Source: CAD feature listing. Evaluate the final solid. Frame: model axes, mm. A direction names the side the tool comes from. Coordinates: 2 decimals unless noted, no trailing zeros. Order: outer loops, then holes, each group sorted by start corner. A loop starts at its lowest first (then second) coordinate and runs counter-clockwise, first axis right, second up.
Item 1: Ray query, line 1 (Y direction, x = -11, z = 0.05); line 2 (X direction, y = 10, z = -1.35); line 3 (Y direction, x = -16.6, z = 0). Return the intervals inside material, ascending.
Item 2: Mould query, pull axis Y, two halves, no side actions, for faces 4 (the cylindrical face through (-8.092, -10.737, 5.917)), 5 (the flat face through (13, 13.5, 0)), 6 (the flat face through (13, -13.5, 0)). Classes: released by +Y, released by -Y, zero draft, split by the parting line, or undercut.
Item 3: Section B-B on y = -3.5. Return the cut outline in (x, z) (3 decimals), then the cut area to 4 significant figures.
Item 4: Contact query for flat-ended pins moving along their axis: P1, Ø4.5, axis at x = 16.5, z = 0, coming from the +Y side; P2, Ø5, axis at x = 9, y = -10, coming from the +Z side (3 decimals); P3, Ø4.5, axis at x = -17, z = 0, coming from the -Y side. Output: stop coordinate, or through.
Item 5: Reachability of faces 1 (the flat face through (-9.1, -13.5, 7.4)), 2 (the flat face through (-4, -2.75, 6)), 3 (the flat face through (18, -4.75, 6)) from +Z, -Z, +X, -X, +Y, -Y: full face, straight path, thin tool, end or side. Return the list, or none.
Item 6: Section A-A on x = 9. Return the cut outline in (y, z) (3 decimals).
Autodesk Inventor part; units mm, degrees
ref_plane "Plan de construction1" through (-9.85, -13.5, 3) normal (0, 0, 1) x (1, 0, 0)
ref_plane "YZ Plane" through (0, 0, 0) normal (1, 0, 0) x (0, 1, 0)
ref_plane "XZ Plane" through (0, 0, 0) normal (0, 1, 0) x (-1, 0, 0)
sketch "Esquisse1" plane through (0, 0, 0) normal (0, 0, 1) x (1, 0, 0)
  line L0 (-21, -13.5) -> (21, -13.5)
  line L1 (21, -13.5) -> (21, 13.5)
  line L2 (21, 13.5) -> (-21, 13.5)
  line L3 (-21, 13.5) -> (-21, -13.5)
  line L4 (-21, -13.5) -> (21, 13.5) construction
  line L5 (21, -13.5) -> (-21, 13.5) construction
  point P0 (0, 0)
  dimension "d0" = 42
  dimension "d1" = 27
extrude "Extrusion1" add sketch "Esquisse1" along normal mid plane 5.75
sketch "Esquisse2" plane through (0, 0, 2.875) normal (0, 0, 1) x (1, 0, 0)
  line L0 (16, -4.75) -> (21, -4.75)
  line L1 (21, -4.75) -> (21, 4)
  line L2 (21, 4) -> (16, 4)
  line L3 (16, 4) -> (16, -4.75)
  line L4 (-21, 6) -> (21, 6)
  line L5 (21, 6) -> (21, 8)
  line L6 (21, 8) -> (-21, 8)
  line L7 (-21, 8) -> (-21, 6)
  line L8 (-21, -4.75) -> (13, -4.75)
  line L9 (13, -4.75) -> (13, -2.75)
  line L10 (13, -2.75) -> (-21, -2.75)
  line L11 (-21, -2.75) -> (-21, -4.75)
  line L12 (-21, -13.5) -> (21, -13.5) construction
  line L13 (21, -13.5) -> (21, 13.5) construction
  line L14 (21, 13.5) -> (-21, 13.5) construction
  line L15 (-21, 13.5) -> (-21, -13.5) construction
  point P0 (0, 0)
  dimension "d4" = 2
  dimension "d5" = 2
  dimension "d6" = 5
  dimension "d7" = 8.75
  dimension "d8" = 2
  dimension "d9" = 5.5
  dimension "d10" = 34
extrude "Extrusion2" add sketch "Esquisse2" along normal blind 6
sketch "Esquisse3" plane through (0, 0, 2.875) normal (0, 0, 1) x (1, 0, 0)
  line L0 (-9.85, 8) -> (7.55, 8)
  line L1 (7.55, 8) -> (7.55, 13.5)
  line L2 (7.55, 13.5) -> (-9.85, 13.5)
  line L3 (-9.85, 13.5) -> (-9.85, 8)
  line L4 (-21, 6) -> (21, 6) construction
  line L5 (21, 6) -> (21, 8) construction
  line L6 (21, 8) -> (-21, 8) construction
  line L7 (-21, 8) -> (-21, 6) construction
  line L8 (-21, 8) -> (21, 8) construction
  line L9 (21, 8) -> (21, 13.5) construction
  line L10 (21, 13.5) -> (-21, 13.5) construction
  line L11 (-21, 13.5) -> (-21, 8) construction
  line L12 (21, 8) -> (-21, 8) construction
  line L13 (-21, -13.5) -> (21, -13.5)
  line L14 (-9.85, -13.5) -> (7.55, -13.5)
  line L15 (7.55, -13.5) -> (7.55, -8.05)
  line L16 (7.55, -8.05) -> (-9.85, -8.05)
  line L17 (-9.85, -8.05) -> (-9.85, -13.5)
  line L18 (-21, -4.75) -> (13, -4.75)
  point P0 (0, 0)
  dimension "d13" = 17.4
  dimension "d14" = 11.15
  dimension "d17" = 3.3
extrude "Extrusion3" add sketch "Esquisse3" along normal up to surface (6 mm away)
ref_plane "Plan de construction1" through (-9.85, -13.5, 3) normal (0, 0, 1) x (1, 0, 0)
sketch "Esquisse5" plane through (-9.85, -13.5, 3) normal (0, 0, 1) x (1, 0, 0)
  line L0 (8.7, 27) -> (8.7, 37.7161)
  line L1 (0, 27) -> (17.4, 27)
  line L2 (0, 27) -> (6.45, 33.5)
  line L3 (6.45, 33.5) -> (8.7, 33.5)
  line L4 (0, 27) -> (8.7, 27)
  line L5 (-11.15, 27) -> (30.85, 27)
  point P0 (9.85, 13.5)
  dimension "d18" = 4.5
  dimension "d19" = 6.5
revolve "Révolution1" add sketch "Esquisse5" angle 360 about axis through (-1.15, 13.5, 3) along (0, 1, 0)
sketch "Esquisse7" plane through (-1.15, 20, 3) normal (0, 1, 0) x (1, 0, 0)
  circle A0 centre (0, 0) radius 2.25 construction
  point P0 (1.15, 3)
hole "Perçage1" at (-1.15, 20, 3) direction (0, -1, 0) diameter 2.459 depth 11 tip angle 118
mirror "Symétrie2" about plane through (0, 0, 0) normal (0, 1, 0) of "Révolution1", "Perçage1"
sketch "Esquisse6" plane through (0, 0, 0) normal (0, 1, 0) x (-1, 0, 0)
  line L0 (7.5667, 8.875) -> (-5.2667, 8.875)
  arc A0 (7.5667, 8.875) -> (-5.2667, 8.875) centre (1.15, 3) ccw
  line L1 (7.5667, -2.875) -> (-5.2667, -2.875)
  arc A1 (-5.2667, -2.875) -> (7.5667, -2.875) centre (1.15, 3) ccw
  point P0 (0, 0)
extrude "Extrusion4" cut sketch "Esquisse6" along normal through all both and the other way through all
sketch "Esquisse8" plane through (-21, -13.5, -2.875) normal (-1, 0, 0) x (0, 0, 1)
  point P0 (2.875, 13.5)
  point P1 (2.875, 13.5)
hole "Perçage2" at (-21, 0, 0) direction (1, 0, 0) diameter 2.459 depth 6 tip angle 118
sketch "Esquisse9" plane through (21, -13.5, -2.875) normal (1, 0, 0) x (0, 0, -1)
  line L0 (-11.75, 8.75) -> (-11.75, 17.5)
  line L1 (-5.75, 17.5) -> (-11.75, 17.5)
  point P0 (-2.875, 13.5)
  point P1 (-8.35, 13.95)
  dimension "d37" = 3.4
  dimension "d38" = 3.55
hole "Perçage3" at (21, 0.45, 5.475) direction (-1, 0, 0) diameter 2.459 end through all
sketch "Esquisse10" plane through (0, 0, -2.875) normal (0, 0, -1) x (-1, 0, 0)
  line L0 (21, -13.5) -> (21, 13.5)
  point P0 (0, 0)
  point P1 (-9, -10)
  point P2 (-9, 10)
  point P3 (11, 10)
  point P4 (11, -10)
  dimension "d46" = 20
  dimension "d47" = 20
  dimension "d48" = 10
  dimension "d49" = 10
hole "Perçage4" at (9, -10, -2.875) at (9, 10, -2.875) at (-11, 10, -2.875) at (-11, -10, -2.875) direction (0, 0, 1) diameter 3 end through all
sketch "Esquisse11" plane through (0, 0, -2.875) normal (0, 0, -1) x (-1, 0, 0)
  line L0 (21, -13.5) -> (21, 13.5)
  line L1 (21, 13.5) -> (7.5667, 13.5)
  point P0 (0, 0)
  point P1 (-5.5, 1.6)
  point P2 (12.75, 1.6)
  dimension "d57" = 18.25
  dimension "d58" = 8.25
  dimension "d59" = 11.9
hole "Perçage5" at (5.5, 1.6, -2.875) at (-12.75, 1.6, -2.875) direction (0, 0, 1) diameter 2.459 end through all
sketch "Esquisse12" plane through (-9.85, -8.05, 8.875) normal (0, 0, 1) x (1, 0, 0)
  arc A0 (17.4, -2.3341) -> (17.4, -1.5659) centre (18.85, -1.95) ccw construction
  arc A1 (0, -0.9869) -> (0, -2.9131) centre (-1.15, -1.95) ccw construction
  arc A2 (0, 19.0131) -> (0, 17.0869) centre (-1.15, 18.05) ccw construction
  arc A3 (17.4, 17.6659) -> (17.4, 18.4341) centre (18.85, 18.05) ccw construction
  circle A4 centre (18.85, -1.95) radius 3
  circle A5 centre (-1.15, -1.95) radius 1.5
  circle A6 centre (-1.15, -1.95) radius 3
  circle A7 centre (-1.15, 18.05) radius 3
  circle A8 centre (18.85, 18.05) radius 1.5
  circle A9 centre (18.85, 18.05) radius 3
  point P0 (9.85, 8.05)
  dimension "d67" = 6
  dimension "d68" = 6
  dimension "d69" = 6
  dimension "d70" = 6
extrude "Extrusion5" cut sketch "Esquisse12" against normal up to surface (6 mm away)
equation "\"d68\" = d67"
equation "\"d69\" = d67"
equation "\"d70\" = d68"
properties part number "Platine" material "Aluminium"
Answer list:
1. line 1: y = -13.5 to -11.5, -8.5 to 8.5, 11.5 to 13.5
1. line 2: x = -21 to -12.5, -9.5 to 7.5, 10.5 to 21
1. line 3: y = -13.5 to -1.23, 1.23 to 13.5
2. face 4: undercut
2. face 5: released by +Y
2. face 6: released by -Y
3. outline: (-21, -2.875) - (21, -2.875) - (21, 8.875) - (16, 8.875) - (16, 2.875) - (13, 2.875) - (13, 8.875) - (-21, 8.875) - close
3. area: 475.5 mm2
4. P1: stops at y = 13.5
4. P2: stops at z = 2.875
4. P3: stops at y = -13.5
5. face 1: +Z, -X, -Y
5. face 2: +Z, -X
5. face 3: +Z, +X, -X, -Y
6. outline: (-13.5, -2.875) - (-11.5, -2.875) - (-11.5, 2.875) - (-13.5, 2.875) - close; (-8.5, -2.875) - (8.5, -2.875) - (8.5, 2.875) - (7, 2.875) - (7, 8.875) - (6, 8.875) - (6, 2.875) - (-2.75, 2.875) - (-2.75, 8.875) - (-4.75, 8.875) - (-4.75, 2.875) - (-8.5, 2.875) - close; (11.5, -2.875) - (13.5, -2.875) - (13.5, 2.875) - (11.5, 2.875) - close
